```python
from build123d import *

# Parameters (mm, degrees)
SKETCH2_R           = 15.875
SKETCH2_R_2         = 12.7
SKETCH2_R_3         = 9.525
BOSS_EXTRUDE1_DEPTH = 3.175
SKETCH3_R           = 1.5875
BOSS_EXTRUDE2_DEPTH = 3.175
CUT_EXTRUDE1_DEPTH  = 3.175


with BuildPart() as part:
    # Sketch2 → Boss-Extrude1 (new body)
    with BuildSketch(Plane.XY):
        Circle(SKETCH2_R)
        Circle(SKETCH2_R_2, mode=Mode.SUBTRACT)
        Circle(SKETCH2_R_2)
        Circle(SKETCH2_R_3, mode=Mode.SUBTRACT)
    extrude(amount=BOSS_EXTRUDE1_DEPTH)

    # Sketch3 → Boss-Extrude2 (add)
    with BuildSketch(Plane.XY.offset(3.175)):
        with BuildLine():
            ThreePointArc((-12.77410023, 9.425390619), (-10.578949158, 11.836446245), (-7.9375, 13.748153285))
            Line((-7.9375, 13.748153285), (-14.2875, 24.746675913))
            Line((-14.2875, 24.746675913), (-19.786761314, 21.571675913))
            Line((-19.786761314, 21.571675913), (-13.436761314, 10.573153285))
            Line((-13.436761314, 10.573153285), (-12.77410023, 9.425390619))
        make_face()
        with Locations((-15.449630657, 20.409545256)):
            Circle(SKETCH3_R, mode=Mode.SUBTRACT)
        with BuildLine():
            Line((14.2875, 24.746675913), (7.9375, 13.748153285))
            ThreePointArc((7.9375, 13.748153285), (10.578949158, 11.836446245), (12.77410023, 9.425390619))
            Line((12.77410023, 9.425390619), (13.436761314, 10.573153285))
            Line((13.436761314, 10.573153285), (19.786761314, 21.571675913))
            Line((19.786761314, 21.571675913), (14.2875, 24.746675913))
        make_face()
        with Locations((15.449630657, 20.409545256)):
            Circle(SKETCH3_R, mode=Mode.SUBTRACT)
    extrude(amount=-BOSS_EXTRUDE2_DEPTH)

    # Sketch5 → Cut-Extrude1 (cut)
    with BuildSketch(Plane.XY.offset(3.175)):
        with BuildLine():
            Line((-7.9375, 13.748153285), (0, 0))
            Line((0, 0), (7.9375, 13.748153285))
            ThreePointArc((7.9375, 13.748153285), (0, 15.875), (-7.9375, 13.748153285))
        make_face()
    extrude(amount=-CUT_EXTRUDE1_DEPTH, mode=Mode.SUBTRACT)


solid = part.part
```
For this review, take the finished solid that the model builds, in its own axes (mm). A direction names the side the tool comes from. Coordinates: 2 decimals unless noted, no trailing zeros. Write each loop counter-clockwise with the first axis right and the second up, starting at its lowest first coordinate (ties: lowest second). Pieces come first, ordered by that corner, then holes. Notation, with made-up numbers: (23, -37.75) -> (82, -37.75) arc R15 ccw to (82, -32.75) -> close; hole circle Ø2 at (8.25, 61.25). An arc over 180 degrees is marked (long way). Put each result on its own line as item: value.
Q1. Clearance check with flat-ended pins moving along their axes: pin 1 Ø5 at (x, y) = (12, -5.5) entering from -Z; pin 2 Ø3 at (x, y) = (-15.45, 20.41) entering from +Z; pin 3 Ø1 at (y, z) = (6, 1) entering from -X. State where each tip first meets the part, or that it passes through.
From the geometry:
pin 1: stops at z = 0
pin 2: passes through
pin 3: stops at x = -14.89
Q2. Tool access review of faces 5 (the flat face through (9.458, 16.382, 1.61)), 6 (the cylindrical face through (-0.49, -15.867, 1.565)): name each direction out of +Z, -Z, +X, -X, +Y, -Y from which nothing blocks a thin tool from reaching the whole face with its end or side.
From the geometry:
face 5: +Z, -Z, +Y
face 6: +Z, -Z
Q3. Take a section at D-D, the plane y = 11.5. State the section outline as (x, z) points (3 decimals).
From the geometry:
outline: (-13.972, 0) -> (-6.64, 0) -> (-6.64, 3.175) -> (-13.972, 3.175) -> close; (6.64, 0) -> (13.972, 0) -> (13.972, 3.175) -> (6.64, 3.175) -> close
Q4. Take a section at A-A, the plane y = 0. State the section outline as (x, z) points (3 decimals), then the cut area to 3 significant figures.
From the geometry:
outline: (-15.875, 0) -> (-9.525, 0) -> (-9.525, 3.175) -> (-15.875, 3.175) -> close; (9.525, 0) -> (15.875, 0) -> (15.875, 3.175) -> (9.525, 3.175) -> close
area: 40.3 mm2
Q5. The part is to be moulded in two halves that separate along Y. For faces 1 (the flat face through (9, 5, 3.175)), 2 (the flat face through (17.076, 23.137, 1.61)), 3 (the cylindrical face through (-0.35, -9.52, 1.57)), 4 (the cylindrical face through (15.11, 18.86, 1.61)), say which applies: +Y half, -Y half, draft (parallel to the pull), parting line (faces both ways), or undercut.
From the geometry:
face 1: draft
face 2: +Y half
face 3: undercut
face 4: undercut
Q6. Take a section at C-C, the plane x = 0. State the section outline as (y, z) points (3 decimals).
From the geometry:
outline: (-15.875, 0) -> (-9.525, 0) -> (-9.525, 3.175) -> (-15.875, 3.175) -> close
Q7. Take a section at B-B, the plane z = 1.9. Count the separate pieces of the cut face and the enclosed holes in it, then the cut area to 3 significant figures.
From the geometry:
separate pieces: 1
enclosed holes: 2
area: 573 mm2
Q8. Wall thickness on L1, parallel to X at y = 20, z = 1.45; L2, parallel to X at y = 21.5, z = 0.1; L3, parallel to Y at x = -14, z = 1.4: over which ranges is each line inside the solid? List them lowest first.
From the geometry:
L1: x = -18.88 to -16.98, -13.92 to -11.55, 11.55 to 13.92, 16.98 to 18.88
L2: x = -19.75 to -16.6, -14.3 to -12.41, 12.41 to 14.3, 16.6 to 19.75
L3: y = -7.48 to 7.48, 11.55 to 19.76, 21.06 to 24.25
